Design review of the part built by this model. Coordinates are the model's own, in mm. Face numbers are marked on the shaded views. A direction names the side the tool comes from. Coordinates: 2 decimals unless noted, no trailing zeros. Loops run counter-clockwise (first coordinate to the right, second up) from the corner with the lowest first, then second, coordinate; pieces in that order, holes last. Notation, with made-up numbers: (-17, -16.5) -> (36, -16.5) arc R29 ccw to (36, 16.5) -> close; hole circle Ø6 at (29.25, -27). An arc over 180 degrees is marked (long way). Use a Markdown table: item, result. Add a question column.
Q1. Take a section at A-A on y = 3.25. Write out the cut boundary in (x, z).
Q2. Clearance check with flat-ended pins moving along their axes: pin 1 Ø10 at (y, z) = (4, 67) entering from +X; pin 2 Ø3 at (y, z) = (7.5, 42.5) entering from +X; pin 3 Ø10 at (y, z) = (1.5, 18) entering from +X. State where each tip first meets the part, or that it passes through.
Q3. Take a section at C-C on z = 6. Write out the cut boundary in (x, y).
Q4. For the marked faces 1 and 2, list the 3-axis set-ups (+Z, -Z, +X, -X, +Y, -Y) from which the entire face can be reached by the end or side of a thin tool; tool diameter is ignored.
Q5. For probe 1 along X at (y, z) = (-6, -8); probe 2 along Z at (x, y) = (5.5, 9.25); probe 3 along X at (y, z) = (2, -20.5), list the stretches that pass through material, from the lowest coordinate up.
Q6. Take a section at B-B on x = 7.5. Write out the cut boundary in (y, z), plus the area to 3 significant figures.
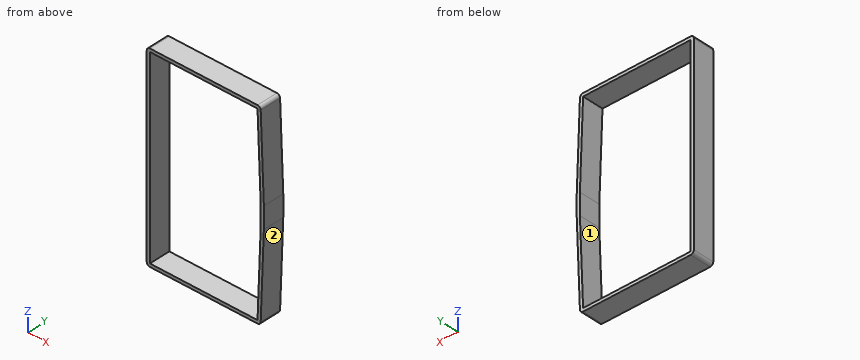
from build123d import *

# Parameters (mm, degrees)
EXTRUDE_THIN1_DEPTH = 10
FILLET1_R           = 3


with BuildPart() as part:
    # Sketch1 → Extrude-Thin1 (new, symmetric)
    with BuildSketch(Plane(origin=(0, 0, 0), x_dir=(1, 0, 0), z_dir=(0, 1, 0))):
        Polygon((57, 10.056230239), (57, -10.056230239), (53.889608634, -93), (-54, -93), (-54, 93), (53.889608634, 93), align=None)
        Polygon((54, 10), (54, -10), (51, -90), (-51, -90), (-51, 90), (51, 90), align=None, mode=Mode.SUBTRACT)
    extrude(amount=EXTRUDE_THIN1_DEPTH, both=True)

    # Fillet1
    fillet1_edges = [part.edges().sort_by_distance(p)[0] for p in [
        (57, 0, 10.056230239),
        (53.889608634, 0, 93),
        (-54, 0, 93),
        (-54, 0, -93),
        (53.889608634, 0, -93),
        (57, 0, -10.056230239),
    ]]
    fillet(fillet1_edges, radius=FILLET1_R)


solid = part.part
Answer list:
| question | item | result |
|---|---|---|
| 1 | outline | (-54, -90) arc R3 ccw to (-51, -93) -> (51, -93) arc R3 ccw to (54, -90.11) -> (57, -10.06) -> (57, 10.06) -> (54, 90.11) arc R3 ccw to (51, 93) -> (-51, 93) arc R3 ccw to (-54, 90) -> close; hole (-51, -90) -> (51, -90) -> (54, -10) -> (54, 10) -> (51, 90) -> (-51, 90) -> close |
| 2 | pin 1 | x = 55.05 |
| 2 | pin 2 | x = 55.84 |
| 2 | pin 3 | x = 56.89 |
| 3 | outline | (-54, -10) -> (-51, -10) -> (-51, 10) -> (-54, 10) -> close; (54, -10) -> (57, -10) -> (57, 10) -> (54, 10) -> close |
| 4 | face 1 | +Y, -Y |
| 4 | face 2 | -Z, +X, +Y, -Y |
| 5 | probe 1 | -54 to -51, 54 to 57 |
| 5 | probe 2 | -93 to -90, 90 to 93 |
| 5 | probe 3 | -54 to -51, 53.61 to 56.61 |
| 6 | outline | (-10, -93) -> (10, -93) -> (10, -90) -> (-10, -90) -> close; (-10, 90) -> (10, 90) -> (10, 93) -> (-10, 93) -> close |
| 6 | area | 120 mm² |
